Work out the finished part from the listing and answer in its coordinate system (mm). Give positions to 0.01 mm unless a question says otherwise; leave off trailing zeros. Order: outer loops, then holes, each group sorted by start corner. A loop starts at its lowest first (then second) coordinate and runs counter-clockwise, first axis right, second up. Notation, with made-up numbers: (2, 31.25) - (21, 31.25) arc R21 cw to (21, 41.25) - close; hole circle Ø2 at (-18, -5.5). An arc over 180 degrees is marked (long way). Return JSON: item names as keys, results as strings. Group by question number.
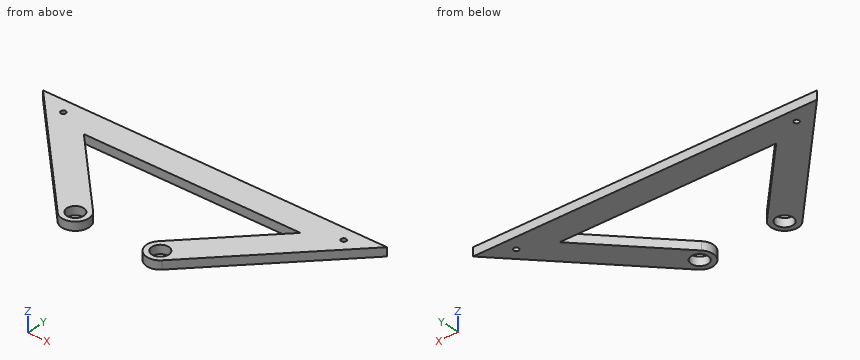
from build123d import *

# Parameters (mm, degrees)
BOSS_EXTRUDE9_DEPTH = 10
SKETCH2_6_R         = 3
SKETCH2_6_R_2       = 10
CUT_EXTRUDE1_DEPTH  = 10
SCALE1_SCALE        = 0.5


with BuildPart() as part:
    # Sketch2 → Boss-Extrude9 (new body)
    with BuildSketch(Plane.XY):
        with BuildLine():
            Line((-127.505639815, 104), (-38.448188718, 11.070485812))
            ThreePointArc((-38.448188718, 11.070485812), (-38.929514188, -11.551811282), (-61.551811282, -11.070485812))
            Line((-61.551811282, -11.070485812), (-202.494360185, 136))
            Line((-202.494360185, 136), (202.494360185, 136))
            Line((202.494360185, 136), (61.551811282, -11.070485812))
            ThreePointArc((61.551811282, -11.070485812), (38.929514188, -11.551811282), (38.448188718, 11.070485812))
            Line((38.448188718, 11.070485812), (127.505639815, 104))
            Line((127.505639815, 104), (-127.505639815, 104))
        make_face()
    extrude(amount=-BOSS_EXTRUDE9_DEPTH)

    # Sketch2<6> → Cut-Extrude1 (cut)
    with BuildSketch(Plane.XY):
        with Locations((-165, 120)):
            Circle(SKETCH2_6_R)
        with Locations((165, 120)):
            Circle(SKETCH2_6_R)
        with Locations((-50, 0)):
            Circle(SKETCH2_6_R_2)
        with Locations((50, 0)):
            Circle(SKETCH2_6_R_2)
    extrude(amount=-CUT_EXTRUDE1_DEPTH, mode=Mode.SUBTRACT)


with BuildPart() as part_1:
    # Scale1: scaled about (0, 89.576748788, -5)
    add(part.part.scale(SCALE1_SCALE).moved(Location((0, 44.788374394, -2.5))))


solid = part_1.part
1. The part is cut by section D-D (x = 51.5). Give the vertices of the cut face in (y, z).
2. Consider probe 1 along Y at (x, z) = (-25, -5.75); probe 2 along Y at (x, z) = (-23, -6); probe 3 along X at (y, z) = (63.5, -4.45). Determine where each line is inside the solid, lowest interval first. Write a range as from..to.
3. The part is cut by section C-C (z = -4.9). Give the vertices of the cut face in (x, y), and give its area (3 significant figures).
4. The part is cut by section A-A (x = -25). Give the vertices of the cut face in (y, z), and give its area (3 significant figures).
5. The part is cut by section B-B (y = 48). Give the vertices of the cut face in (x, z), and give its area (3 significant figures).
6. Each of these flat-tipped pins is pushed along its axis until it touches: pin 1 (8 mm diameter, centred on x = 71, y = 73.5, fed in from -Z); pin 2 (2 mm diameter, centred on y = 95, z = -3.5, fed in from +X); pin 3 (1.5 mm diameter, centred on y = 103, z = -6, fed in from +X). Where does it stop, or does it pass through?
Answers:
{
 "1": {"outline": "(60.88, -7.5) - (84, -7.5) - (84, -2.5) - (60.88, -2.5) - close; (96.79, -7.5) - (112.79, -7.5) - (112.79, -2.5) - (96.79, -2.5) - close"},
 "2": {"probe 1": "y = 36.79..39.79, 49.79..56.35, 96.79..112.79", "probe 2": "y = 37.04..40.21, 49.37..54.26, 96.79..112.79", "probe 3": "x = -54.01..-31.85, 31.85..54.01"},
 "3": {"outline": "(-101.25, 112.79) - (-30.78, 39.25) arc R8 ccw to (-19.22, 50.32) - (-63.75, 96.79) - (63.75, 96.79) - (19.22, 50.32) arc R8 ccw to (30.78, 39.25) - (101.25, 112.79) - close; hole circle Ø3 at (-82.5, 104.79); hole circle Ø10 at (-25, 44.79); hole circle Ø10 at (25, 44.79); hole circle Ø3 at (82.5, 104.79)", "area": "5,330 mm^2"},
 "4": {"outline": "(36.79, -7.5) - (39.79, -7.5) - (39.79, -2.5) - (36.79, -2.5) - close; (49.79, -7.5) - (56.35, -7.5) - (56.35, -2.5) - (49.79, -2.5) - close; (96.79, -7.5) - (112.79, -7.5) - (112.79, -2.5) - (96.79, -2.5) - close", "area": "128 mm^2"},
 "5": {"outline": "(-39.16, -7.5) - (-28.83, -7.5) - (-28.83, -2.5) - (-39.16, -2.5) - close; (-21.17, -7.5) - (-17.67, -7.5) - (-17.67, -2.5) - (-21.17, -2.5) - close; (17.67, -7.5) - (21.17, -7.5) - (21.17, -2.5) - (17.67, -2.5) - close; (28.83, -7.5) - (39.16, -7.5) - (39.16, -2.5) - (28.83, -2.5) - close", "area": "138 mm^2"},
 "6": {"pin 1": "passes through", "pin 2": "stops at x = 85.16", "pin 3": "stops at x = 92.59"}
}
